Geometry: final body of the model. Coordinates: model frame, mm. A direction names the side the tool comes from. Round coordinates to 2 decimals unless told otherwise and drop trailing zeros. Loops run counter-clockwise (first coordinate to the right, second up) from the corner with the lowest first, then second, coordinate; pieces in that order, holes last. Notation, with made-up numbers: M 18,41 L 77,41 A16 ccw 77,55 Z; hole C 51,-23 d8. An arc over 180 degrees is marked long. Answer as a JSON object with one key per item and string values.
from build123d import *

# Parameters (mm, degrees)
SKETCH1_R               = 22.5
BOSS_EXTRUDE1_DEPTH     = 5.91
SKETCH2_R               = 6
BOSS_EXTRUDE2_DEPTH     = 200
SKETCH3_R               = 12
BOSS_EXTRUDE3_DEPTH     = 28
FILLET1_R               = 6
CUT_EXTRUDE1_DEPTH      = 209.354093072
CUT_EXTRUDE1_DEPTH_BACK = 209.354093072
SKETCH4_W               = 21.071752118
SKETCH4_H               = 26
SKETCH5_R               = 7.5
CUT_EXTRUDE2_DEPTH      = 209.953172027


with BuildPart() as part:
    # Sketch1 → Boss-Extrude1 (new body)
    with BuildSketch(Plane.XY):
        Circle(SKETCH1_R)
    extrude(amount=BOSS_EXTRUDE1_DEPTH)

    # Sketch2 → Boss-Extrude2 (add)
    with BuildSketch(Plane.XY.offset(5.91)):
        Circle(SKETCH2_R)
    extrude(amount=BOSS_EXTRUDE2_DEPTH)

    # Sketch3 → Boss-Extrude3 (add)
    with BuildSketch(Plane(origin=(0, 0, 0), x_dir=(-1, 0, 0), z_dir=(0, 0, -1))):
        with Locations(Location((0, 0, 0), (0, 0, 180))):
            Circle(SKETCH3_R)
    extrude(amount=BOSS_EXTRUDE3_DEPTH)

    # Fillet1
    fillet1_edges = [part.edges().sort_by_distance(p)[0] for p in [
        (-12, 0, -28),
    ]]
    fillet(fillet1_edges, radius=FILLET1_R)

    # Sketch4 → Cut-Extrude1 (cut, two sides: drawn at the far end of the back side and taken through both)
    with BuildSketch(Plane(origin=(0, 0, 0), x_dir=(1, 0, 0), z_dir=(0, 1, 0)).offset(-CUT_EXTRUDE1_DEPTH_BACK)):
        with Locations((-15.535876059, 16)):
            Rectangle(SKETCH4_W, SKETCH4_H)
        with Locations((15.535876059, 16)):
            Rectangle(SKETCH4_W, SKETCH4_H)
    extrude(amount=CUT_EXTRUDE1_DEPTH + CUT_EXTRUDE1_DEPTH_BACK, mode=Mode.SUBTRACT)

    # Sketch5 → Cut-Extrude2 (cut, through all)
    with BuildSketch(Plane(origin=(5, 0, 0), x_dir=(0, 0, -1), z_dir=(1, 0, 0))):
        with Locations((15.5, 0)):
            Circle(SKETCH5_R)
    extrude(amount=-CUT_EXTRUDE2_DEPTH, mode=Mode.SUBTRACT)


solid = part.part
1) Section query D-D (x = 14.5). Return the cut outline in (y, z).
Results:
{"outline": "M -17.2,0 L 17.2,0 L 17.2,5.91 L -17.2,5.91 Z"}
2) Pull-direction query (Y, two-part tool) for faces 1 (the cylindrical face through (0, 0, -8)), 2 (the cylindrical face through (-4.591, -11.087, -8.504)), 3 (the flat face through (10, -10, 0)); classes: +Y half, -Y half, draft (parallel to the pull), parting line (faces both ways), or undercut.
Results:
{"face 1": "undercut", "face 2": "parting line", "face 3": "draft"}
3) Pin query (flat end, axial travel): P1, Ø8, axis at x = 8.5, y = -14, coming from the -Z side; P2, Ø12, axis at y = 0, z = -15.5, coming from the +X side; P3, Ø3.5, axis at x = -9, y = 4, coming from the -Z side; P4, Ø1.5, axis at x = 1.5, z = 121.5, coming from the +Y side. Return the tip coordinate at first contact, or that it passes through.
Results:
{"P1": "z = 0", "P2": "through", "P3": "z = -3", "P4": "y = 5.95"}
4) Section query C-C (z = 184). Return the cut outline in (x, y).
Results:
{"outline": "C 0,0 d12"}
5) Reachability of faces 4 (the flat face through (-8, 0, -3)), 5 (the flat face through (0, 0, 205.91)), 6 (the flat face through (8, 0, -3)), 7 (the flat face through (0, 0, -28)), 8 (the flat face through (5, -5, 5.91)) from +Z, -Z, +X, -X, +Y, -Y: full face, straight path, thin tool, end or side. Return the list, or none.
Results:
{"face 4": "-Z, -X, +Y, -Y", "face 5": "+Z, +X, -X, +Y, -Y", "face 6": "-Z, +X, +Y, -Y", "face 7": "-Z, +X, -X, +Y, -Y", "face 8": "+Z"}
6) Section query B-B (y = 0). Return the cut outline in (x, z), and give its area (3 significant figures).
Results:
{"outline": "M -22.5,0 L -12,0 L -12,-3 L -5,-3 L -5,-8 L 5,-8 L 5,-3 L 12,-3 L 12,0 L 22.5,0 L 22.5,5.91 L 6,5.91 L 6,205.91 L -6,205.91 L -6,5.91 L -22.5,5.91 Z; M -5,-28 L 5,-28 L 5,-23 L -5,-23 Z", "area": "2,840 mm2"}
7) Ray query, line 1 (Y direction, x = -0.25, z = -15.5); line 2 (Z direction, x = -9.5, y = 4.5); line 3 (Y direction, x = 2, z = -15). Return the intervals inside material, ascending.
Results:
{"line 1": "-12 to -7.5, 7.5 to 12", "line 2": "-3 to 5.91", "line 3": "-11.83 to -7.48, 7.48 to 11.83"}
8) Section query A-A (z = -15.5). Return the cut outline in (x, y).
Results:
{"outline": "M -5,-10.91 A12 ccw 5,-10.91 L 5,-7.5 L -5,-7.5 Z; M -5,7.5 L 5,7.5 L 5,10.91 A12 ccw -5,10.91 Z"}
